```python
from build123d import *

# Parameters (mm, degrees)
BOSS_EXTRUDE1_DEPTH      = 0.8
BOSS_EXTRUDE2_DEPTH      = 8.509
CUT_EXTRUDE1_DEPTH       = 8.509
X_0_397_DIAMETER_HOLE1_D = 3.099999896
SKETCH8_W                = 23.81809924
SKETCH8_H                = 9.191548364
BOSS_EXTRUDE4_DEPTH      = 5


with BuildPart() as part:
    # Sketch1 → Boss-Extrude1 (new body)
    with BuildSketch(Plane(origin=(0, 0, 0), x_dir=(0, 0, -1), z_dir=(1, 0, 0))):
        with BuildLine():
            Line((-17.08, -6.275), (17.08, -6.275))
            ThreePointArc((17.08, -6.275), (18.876051224, -5.531051224), (19.62, -3.735))
            Line((19.62, -3.735), (19.62, 3.735))
            ThreePointArc((19.62, 3.735), (18.876051224, 5.531051224), (17.08, 6.275))
            Line((17.08, 6.275), (-17.08, 6.275))
            ThreePointArc((-17.08, 6.275), (-18.876051224, 5.531051224), (-19.62, 3.735))
            Line((-19.62, 3.735), (-19.62, -3.735))
            ThreePointArc((-19.62, -3.735), (-18.876051224, -5.531051224), (-17.08, -6.275))
        make_face()
    extrude(amount=BOSS_EXTRUDE1_DEPTH)

    # Sketch2 → Boss-Extrude2 (add)
    with BuildSketch(Plane(origin=(0.8, 0, 0), x_dir=(0, 0, -1), z_dir=(1, 0, 0))):
        with BuildLine():
            Line((-9.314807553, 5.005), (9.314807553, 5.005))
            ThreePointArc((9.314807553, 5.005), (11.329925037, 4.01125403), (11.768259152, 1.807599625))
            Line((11.768259152, 1.807599625), (10.447269633, -3.122400375))
            ThreePointArc((10.447269633, -3.122400375), (9.540072064, -4.480117484), (7.993818034, -5.005))
            Line((7.993818034, -5.005), (-7.993818034, -5.005))
            ThreePointArc((-7.993818034, -5.005), (-9.540072064, -4.480117484), (-10.447269633, -3.122400375))
            Line((-10.447269633, -3.122400375), (-11.768259152, 1.807599625))
            ThreePointArc((-11.768259152, 1.807599625), (-11.329925037, 4.01125403), (-9.314807553, 5.005))
        make_face()
    extrude(amount=BOSS_EXTRUDE2_DEPTH)

    # Sketch3 → Cut-Extrude1 (cut)
    with BuildSketch(Plane(origin=(9.309, 0, 0), x_dir=(0, 0, -1), z_dir=(1, 0, 0))):
        with BuildLine():
            Line((-11.032223672, 2.004819738), (-9.711234153, -2.925180262))
            ThreePointArc((-9.711234153, -2.925180262), (-9.076195855, -3.875582239), (-7.993818034, -4.243))
            Line((-7.993818034, -4.243), (7.993818034, -4.243))
            ThreePointArc((7.993818034, -4.243), (9.076195855, -3.875582239), (9.711234153, -2.925180262))
            Line((9.711234153, -2.925180262), (11.032223672, 2.004819738))
            ThreePointArc((11.032223672, 2.004819738), (10.725389792, 3.547377821), (9.314807553, 4.243))
            Line((9.314807553, 4.243), (-9.314807553, 4.243))
            ThreePointArc((-9.314807553, 4.243), (-10.725389792, 3.547377821), (-11.032223672, 2.004819738))
        make_face()
    extrude(amount=-CUT_EXTRUDE1_DEPTH, mode=Mode.SUBTRACT)

    # X (0.397) Diameter Hole1 (through all)
    with Locations(Plane(origin=(0.8, 0, 0), x_dir=(0, 0, -1), z_dir=(1, 0, 0))):
        with Locations((-16.66, 0), (16.66, 0)):
            Hole(X_0_397_DIAMETER_HOLE1_D / 2)

    # Sketch8 → Boss-Extrude4 (add)
    with BuildSketch(Plane.ZY):
        Rectangle(SKETCH8_W, SKETCH8_H)
    extrude(amount=BOSS_EXTRUDE4_DEPTH)


solid = part.part
```
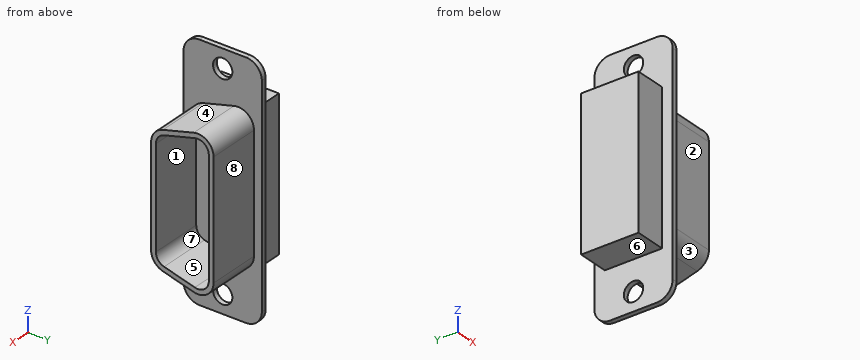
Build history of the part. All positions in model axes, mm. Face numbers are marked on the shaded views. A direction names the side the tool comes from. Coordinates: 2 decimals unless noted, no trailing zeros. Order: outer loops, then holes, each group sorted by start corner. A loop starts at its lowest first (then second) coordinate and runs counter-clockwise, first axis right, second up.
Item 1: Tool access for the marked faces 1, 2, 3 and 4: list every direction of +Z, -Z, +X, -X, +Y, -Y with a clear straight run to the whole face (end or side of a thin tool).
Filled in:
face 1: +X
face 2: +Z, -Z, +X, -Y
face 3: -Z, +X, -Y
face 4: +Z, +X, -Y
Item 2: Saw through at A-A on z = 16.66. List the corners of the cut face in (x, y) (3 decimals), then the cut area to 3 significant figures.
Filled in:
outline: (0, -6.275) - (0.8, -6.275) - (0.8, -1.55) - (0, -1.55) - close; (0, 1.55) - (0.8, 1.55) - (0.8, 6.275) - (0, 6.275) - close
area: 7.56 mm2
Item 3: Saw through at B-B on y = 0. List the corners of the cut face in (x, z), then the cut area to 3 significant figures.
Filled in:
outline: (-5, -11.91) - (0, -11.91) - (0, -15.11) - (0.8, -15.11) - (0.8, -11.28) - (9.31, -11.28) - (9.31, -10.5) - (0.8, -10.5) - (0.8, 10.5) - (9.31, 10.5) - (9.31, 11.28) - (0.8, 11.28) - (0.8, 15.11) - (0, 15.11) - (0, 11.91) - (-5, 11.91) - close; (0, -19.62) - (0.8, -19.62) - (0.8, -18.21) - (0, -18.21) - close; (0, 18.21) - (0.8, 18.21) - (0.8, 19.62) - (0, 19.62) - close
area: 159 mm2
Item 4: Drop flat-ended pins along their axis: pin 1 Ø2.5 at (x, z) = (4.5, -1.5) entering from +Y (3 decimals); pin 2 Ø4 at (x, y) = (2.5, -3) entering from +Z; pin 3 Ø2.5 at (x, z) = (-3, 1) entering from -Y; pin 4 Ø1.5 at (y, z) = (-1, 6.5) entering from +X. Give the stop position or say it passes through.
Filled in:
pin 1: stops at y = 5.005
pin 2: stops at z = 19.62
pin 3: stops at y = -4.6
pin 4: stops at x = 0.8
Item 5: Saw through at D-D on y = -2.25. List the corners of the cut face in (x, z).
Filled in:
outline: (-5, -11.91) - (0, -11.91) - (0, -19.62) - (0.8, -19.62) - (0.8, -10.68) - (9.31, -10.68) - (9.31, -9.89) - (0.8, -9.89) - (0.8, 9.89) - (9.31, 9.89) - (9.31, 10.68) - (0.8, 10.68) - (0.8, 19.62) - (0, 19.62) - (0, 11.91) - (-5, 11.91) - close
Item 6: Mould opens along Z. For the marked faces 5, 6, 7 and 8 say: released by +Z, released by -Z, zero draft, split by the parting line, or undercut.
Filled in:
face 5: undercut
face 6: released by -Z
face 7: undercut
face 8: zero draft
Item 7: Saw through at C-C on z = -5. List the corners of the cut face in (x, y) (3 decimals).
Filled in:
outline: (-5, -4.596) - (0, -4.596) - (0, -6.275) - (0.8, -6.275) - (0.8, -5.005) - (9.309, -5.005) - (9.309, -4.243) - (0.8, -4.243) - (0.8, 4.243) - (9.309, 4.243) - (9.309, 5.005) - (0.8, 5.005) - (0.8, 6.275) - (0, 6.275) - (0, 4.596) - (-5, 4.596) - close
Item 8: Drill centre lines: L1, parallel to Y at x = 1.5, z = -0.5 (3 decimals); L2, parallel to Y at x = 0.6, z = 16.66 (3 decimals); L3, parallel to X at y = -1.5, z = 17.5. Where is each one in solid material? Low to high.
Filled in:
L1: y = -5.005 to -4.243, 4.243 to 5.005
L2: y = -6.275 to -1.55, 1.55 to 6.275
L3: x = 0 to 0.8
